Build history of the part. All positions in model axes, mm. A direction names the side the tool comes from. Round coordinates to 2 decimals unless told otherwise and drop trailing zeros. Loops run counter-clockwise (first coordinate to the right, second up) from the corner with the lowest first, then second, coordinate; pieces in that order, holes last. Notation, with made-up numbers: (-14.75, -23) -> (14.25, -23) arc R6 cw to (14.25, -15) -> close; hole circle Ø3 at (-37, -1). An arc over 180 degrees is marked (long way). Put each result on its own line as item: value. Start each with the question number.
```python
from build123d import *

# Parameters (mm, degrees)
SKETCH1_W           = 42
SKETCH1_H           = 42
BOSS_EXTRUDE1_DEPTH = 48
SKETCH2_R           = 4
BOSS_EXTRUDE2_DEPTH = 310
FILLET1_R           = 2.54


with BuildPart() as part:
    # Sketch1 → Boss-Extrude1 (new body)
    with BuildSketch(Plane(origin=(0, 0, 0), x_dir=(1, 0, 0), z_dir=(0, 1, 0))):
        Rectangle(SKETCH1_W, SKETCH1_H)
    extrude(amount=BOSS_EXTRUDE1_DEPTH)

    # Sketch2 → Boss-Extrude2 (add)
    with BuildSketch(Plane(origin=(0, 48, 0), x_dir=(1, 0, 0), z_dir=(0, 1, 0))):
        with Locations(Location((0, 0, 0), (0, 0, 90))):
            Circle(SKETCH2_R)
    extrude(amount=BOSS_EXTRUDE2_DEPTH)

    # Fillet1
    fillet1_edges = [part.edges().sort_by_distance(p)[0] for p in [
        (-21, 48, 0),
        (0, 48, 21),
        (21, 48, 0),
        (0, 0, 21),
        (-21, 0, 0),
        (0, 0, -21),
        (21, 0, 0),
        (0, 48, -21),
        (21, 24, 21),
        (-21, 24, 21),
        (-21, 24, -21),
        (21, 24, -21),
    ]]
    fillet(fillet1_edges, radius=FILLET1_R)


solid = part.part
```
Item 1: Cut at B-B on z = 0. Write the cut outline in (x, y), then the cut area to 3 significant figures.
Item 2: Wall check: line 1 (Y direction, x = -17, z = 16.5); line 2 (Y direction, x = -18.5, z = -19); line 3 (X direction, y = 218.5, z = 2.5). Give the ranges that are in metal, low to high. Write a range as from..to.
Item 3: Cut at D-D on x = 15.5. Write the cut outline in (y, z), then the cut area to 3 significant figures.
Item 4: Drop flat-ended pins along their axis: pin 1 (5 mm diameter, centred on x = -5.5, y = 132, fed in from +Z); pin 2 (5 mm diameter, centred on y = 266, z = -8.5, fed in from +X); pin 3 (3 mm diameter, centred on x = -2.5, y = 192, fed in from -Z); pin 4 (8 mm diameter, centred on y = 186.5, z = 3, fed in from -X). Give the stop position or say it passes through.
Item 5: Cut at C-C on y = 312.5. Write the cut outline in (x, z), then the cut area to 3 significant figures.
Item 6: 3-axis set-ups, long thin cutter, end or side, ignore diameter. For faces 1 (the face through (3.905, 200.83, 0.867)), 2 (the face through (0, 358, 0)): which of +Z, -Z, +X, -X, +Y, -Y reach the whole face in a straight line?
Item 7: Cut at A-A on x = 0. Write the cut outline in (y, z), then the cut area to 3 significant figures.
Ans:
1. outline: (-21, 2.54) arc R2.54 ccw to (-18.46, 0) -> (18.46, 0) arc R2.54 ccw to (21, 2.54) -> (21, 45.46) arc R2.54 ccw to (18.46, 48) -> (4, 48) -> (4, 358) -> (-4, 358) -> (-4, 48) -> (-18.46, 48) arc R2.54 ccw to (-21, 45.46) -> close
1. area: 4,490 mm2
2. line 1: y = 0..48
2. line 2: y = 0.06..47.94
2. line 3: x = -3.12..3.12
3. outline: (0, -18.46) arc R2.54 ccw to (2.54, -21) -> (45.46, -21) arc R2.54 ccw to (48, -18.46) -> (48, 18.46) arc R2.54 ccw to (45.46, 21) -> (2.54, 21) arc R2.54 ccw to (0, 18.46) -> close
3. area: 2,010 mm2
4. pin 1: stops at z = 2.65
4. pin 2: passes through
4. pin 3: stops at z = -3.87
4. pin 4: stops at x = -4
5. outline: circle Ø8 at (0, 0)
5. area: 50.3 mm2
6. face 1: +Y
6. face 2: +Z, -Z, +X, -X, +Y
7. outline: (0, -18.46) arc R2.54 ccw to (2.54, -21) -> (45.46, -21) arc R2.54 ccw to (48, -18.46) -> (48, -4) -> (358, -4) -> (358, 4) -> (48, 4) -> (48, 18.46) arc R2.54 ccw to (45.46, 21) -> (2.54, 21) arc R2.54 ccw to (0, 18.46) -> close
7. area: 4,490 mm2
